```python
from build123d import *

# Parameters (mm, degrees)
F3_W           = 8.3933982822
F3_H           = 16.3933982822
F4_ANGLE_BACK  = 70
F4_ANGLE       = 140
F6_ANGLE_START = 100
F6_ANGLE       = 160
F7_ANGLE_BACK  = 70
F7_ANGLE       = 140
F8_R           = 3
F8_2_R         = 3
F9_R           = 3


with BuildPart() as f1:
    # F0 (on Front) → F1 (revolve)
    with BuildSketch(Plane.XZ):
        Polygon((-44, 15), (-27, -2), (0, -2), (0, 20), (-44, 20), align=None)
    revolve(axis=Axis((0, 0, 9.4880101401), (0, 0, -1)))


with BuildPart() as f4:
    # F3 (on Front) → F4 (revolve)
    with BuildSketch(Plane.XZ, mode=Mode.PRIVATE) as f4_sk:
        with Locations((-41.8033008589, 16.8033008589)):
            Rectangle(F3_W, F3_H)
    revolve(f4_sk.sketch.rotate(Axis((0, 0, 9.4880101401), (0, 0, -1)), -F4_ANGLE_BACK), axis=Axis((0, 0, 9.4880101401), (0, 0, -1)), revolution_arc=F4_ANGLE)

    # F8#2
    f8_2_edges = [f4.edges().sort_by_distance(p)[0] for p in [
        (-12.862215, 35.338646, 16.803301),
        (-12.862215, -35.338646, 16.803301),
    ]]
    fillet(f8_2_edges, radius=F8_2_R)


with BuildPart() as f6:
    # F5 (on Front) → F6 (revolve)
    with BuildSketch(Plane.XZ, mode=Mode.PRIVATE) as f6_sk:
        Polygon((-36.8994949366, -6.2426406871), (-25.5857864376, 5.0710678119), (-37.6066017178, 17.091883092), (-48.9203102168, 5.7781745931), align=None)
    revolve(f6_sk.sketch.rotate(Axis((0, 0, 9), (0, 0, -1)), F6_ANGLE_START), axis=Axis((0, 0, 9), (0, 0, -1)), revolution_arc=F6_ANGLE)

    # F9
    f9_edges = [f6.edges().sort_by_distance(p)[0] for p in [
        (5.425228, 30.767995, -0.585786),
        (7.51262, 42.606187, 11.435029),
        (7.51262, -42.606187, 11.435029),
        (5.425228, -30.767995, -0.585786),
    ]]
    fillet(f9_edges, radius=F9_R)


with BuildPart() as f7:
    # F2 (on Front) → F7 (revolve)
    with BuildSketch(Plane.XZ, mode=Mode.PRIVATE) as f7_sk:
        Polygon((-42.7019295049, 3.5112739307), (-33.3639610307, 12.8492424049), (-37.6066017178, 17.091883092), (-46.944570192, 7.7539146178), align=None)
    revolve(f7_sk.sketch.rotate(Axis((0, 0, 9), (0, 0, -1)), -F7_ANGLE_BACK), axis=Axis((0, 0, 9), (0, 0, -1)), revolution_arc=F7_ANGLE)

    # F8
    f8_edges = [f7.edges().sort_by_distance(p)[0] for p in [
        (-13.008033, -35.739278, 8.180258),
        (-13.008033, 35.739278, 8.180258),
    ]]
    fillet(f8_edges, radius=F8_R)


with BuildPart() as f1_1:
    add(f1.part)

    # F10: cut F7, F4, F6
    add(f7.part, mode=Mode.SUBTRACT)
    add(f4.part, mode=Mode.SUBTRACT)
    add(f6.part, mode=Mode.SUBTRACT)


solid = f1_1.part
```
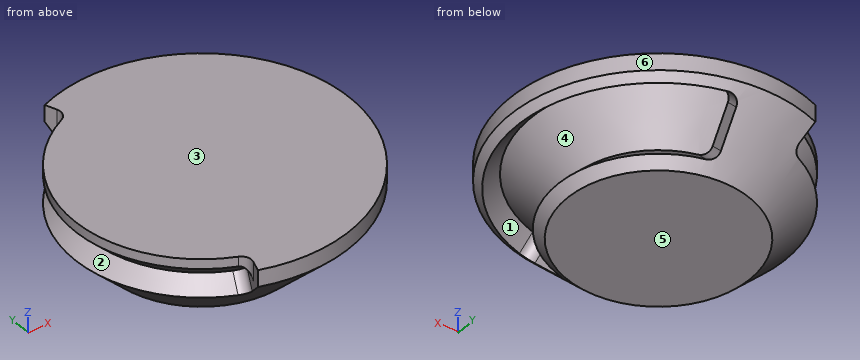
Design review of the part built by this model. Coordinates are the model's own, in mm. Face numbers are marked on the shaded views. A direction names the side the tool comes from. Round coordinates to 2 decimals unless told otherwise and drop trailing zeros. Write each loop counter-clockwise with the first axis right and the second up, starting at its lowest first coordinate (ties: lowest second). Pieces come first, ordered by that corner, then holes.
Item 1: For probe 1 along Y at (x, z) = (29.5, 15); probe 2 along Y at (x, z) = (12, 15); probe 3 along X at (y, z) = (12, 15.25), list the stretches that pass through material, from the lowest coordinate up.
Item 2: We need section A-A on x = 0. Write out the cut boundary in (y, z).
Item 3: Clearance check with flat-ended pins moving along their axes: pin 1 Ø2 at (x, z) = (3, 11.5) entering from +Y; pin 2 Ø6 at (y, z) = (-3.5, 11.5) entering from +X; pin 3 Ø4 at (x, z) = (3.5, 7.5) entering from +Y. State where each tip first meets the part, or that it passes through.
Item 4: For the marked faces 1, 2 and 3, list the 3-axis set-ups (+Z, -Z, +X, -X, +Y, -Y) from which the entire face can be reached by the end or side of a thin tool; tool diameter is ignored.
Item 5: We need section C-C on z = 18.5. Write out the cut boundary in (x, y).
Item 6: The part is to be moulded in two halves that separate along Y. For the marked faces 4, 5 and 6, say which applies: +Y half, -Y half, draft (parallel to the pull), parting line (faces both ways), or undercut.
Item 7: We need section B-B on y = 0. Write out the cut boundary in (x, z), and give its area (3 significant figures).
Returned:
1. probe 1: y = -32.65 to -26.57, -19.77 to 19.77, 26.57 to 32.65
1. probe 2: y = -42.33 to -37.84, -33.43 to 33.43, 37.84 to 42.33
1. probe 3: x = -33.69 to 33.69, 37.58 to 42.33
2. outline: (-44, 15) - (-27, -2) - (27, -2) - (44, 15) - (44, 20) - (-44, 20) - close
3. pin 1: stops at y = 41.39
3. pin 2: stops at x = 43.37
3. pin 3: stops at y = 38.35
4. face 1: -Z
4. face 2: -X
4. face 3: +Z, +X, -X, +Y, -Y
5. outline: (-15.44, -34.29) arc R3 cw to (-13.85, -38.05) - (-15.05, -41.35) arc R44 ccw (long way) to (-15.05, 41.35) - (-13.85, 38.05) arc R3 cw to (-15.44, 34.29) arc R37.61 ccw to start
6. face 4: undercut
6. face 5: draft
6. face 6: parting line
7. outline: (-37.61, 8.61) - (-27, -2) - (27, -2) - (29.83, 0.83) - (25.59, 5.07) - (37.61, 17.09) - (41.85, 12.85) - (44, 15) - (44, 20) - (-37.61, 20) - (-37.61, 17.09) - (-33.36, 12.85) - close
7. area: 1,470 mm2
